from build123d import *

# Parameters (mm, degrees)
EXTRUDE_1_DEPTH         = 4
HOLE_WIZARD_5_5_5_5_2_D = 5.5
HOLE_WIZARD_5_5_5_5_1_D = 5.5
HOLE_WIZARD_6_6_6_6_1_D = 6.6
CUT_EXTRUDE_1_DEPTH     = 5


with BuildPart() as part:
    # Эскиз1 → Бобышка-Вытянуть1 (new body)
    with BuildSketch(Plane(origin=(0, 0, 0), x_dir=(1, 0, 0), z_dir=(0, 1, 0))):
        Polygon((0, 386), (74.75, 386), (74.75, 382), (105.25, 382), (105.25, 386), (180, 386), (180, 0), (0, 0), align=None)
    extrude(amount=EXTRUDE_1_DEPTH)

    # Диаметр отверстия Ø5.5 (5.5)2 (through all)
    with Locations(Plane(origin=(0, 4, 0), x_dir=(1, 0, 0), z_dir=(0, 1, 0))):
        with Locations((78, 238), (78, 278), (102, 238), (102, 278), (128, 174), (128, 142), (98, 142), (98, 174), (128, 374), (98, 374), (128, 342), (98, 342), (52, 174), (52, 142), (82, 142), (82, 174), (52, 342), (82, 342), (52, 374), (82, 374)):
            Hole(HOLE_WIZARD_5_5_5_5_2_D / 2)

    # Диаметр отверстия Ø5.5 (5.5)1 (through all)
    with Locations(Plane(origin=(0, 4, 0), x_dir=(1, 0, 0), z_dir=(0, 1, 0))):
        with Locations((8, 75), (8, 225), (172, 225), (172, 75), (38, 225), (38, 75), (142, 225), (142, 75)):
            Hole(HOLE_WIZARD_5_5_5_5_1_D / 2)

    # Диаметр отверстия Ø6.6 (6.6)1 (through all)
    with Locations(Plane(origin=(0, 4, 0), x_dir=(1, 0, 0), z_dir=(0, 1, 0))):
        with Locations((67, 327), (113, 327), (67, 314), (113, 314)):
            Hole(HOLE_WIZARD_6_6_6_6_1_D / 2)

    # Эскиз8 → Вырез-Вытянуть1 (cut, through all)
    with BuildSketch(Plane(origin=(0, 4, 0), x_dir=(1, 0, 0), z_dir=(0, 1, 0))):
        with BuildLine():
            Line((70.3, 24.5), (70.3, 14.5))
            ThreePointArc((70.3, 14.5), (67, 11.2), (63.7, 14.5))
            Line((63.7, 14.5), (63.7, 24.5))
            ThreePointArc((63.7, 24.5), (67, 27.8), (70.3, 24.5))
        make_face()
        with BuildLine():
            Line((109.7, 14.5), (109.7, 24.5))
            ThreePointArc((109.7, 24.5), (113, 27.8), (116.3, 24.5))
            Line((116.3, 24.5), (116.3, 14.5))
            ThreePointArc((116.3, 14.5), (113, 11.2), (109.7, 14.5))
        make_face()
    extrude(amount=-CUT_EXTRUDE_1_DEPTH, mode=Mode.SUBTRACT)


solid = part.part
The model under review builds one solid part; all positions refer to its coordinate system, in mm. Coordinates: 2 decimals unless noted, no trailing zeros. Answer in a Markdown table with one row per item.
1. We need section A-A, the plane y = 1.8. Give the number of separate pieces and of enclosed holes in the cut face, and give its area (3 significant figures).
Answers below:
| item | result |
|---|---|
| separate pieces | 1 |
| enclosed holes | 34 |
| area | 68,400 mm^2 |
2. Draft analysis for pull direction Z (two halves, no side actions). For faces 1 (the flat face through (91, 4, -196)), 2 (the cylindrical face through (65.48, 1.97, -311.07)), 3 (the cylindrical face through (113.72, 1.97, -310.78)), state which applies: +Z half, -Z half, draft (parallel to the pull), parting line (faces both ways), or undercut.
Answers below:
| item | result |
|---|---|
| face 1 | draft |
| face 2 | undercut |
| face 3 | undercut |
3. Wall thickness on probe 1 along X at (y, z) = (1.9, -225); probe 2 along X at (y, z) = (3.05, -238); probe 3 along Z at (x, y) = (82, 1.9): over which ranges is each line inside the solid? List them lowest first. Write a range as [from, to].
Answers below:
| item | result |
|---|---|
| probe 1 | x = [0, 5.25], [10.75, 35.25], [40.75, 139.25], [144.75, 169.25], [174.75, 180] |
| probe 2 | x = [0, 75.25], [80.75, 99.25], [104.75, 180] |
| probe 3 | z = [-382, -376.75], [-371.25, -344.75], [-339.25, -176.75], [-171.25, -144.75], [-139.25, 0] |
